from build123d import *


with BuildPart() as part:
    # Эскиз1 → Повернуть1 (revolve)
    with BuildSketch(Plane(origin=(0, 0, 0), x_dir=(1, 0, 0), z_dir=(0, 1, 0)), mode=Mode.PRIVATE) as revolve_1_sk:
        Polygon((5.5, 5), (5.5, 6), (4.5, 6), (4.5, 7), (3.5, 7), (3.5, 8), (6, 8), (6, 10), (3, 10), (3, -10), (6, -10), (6, -8), (3.5, -8), (3.5, -7), (4.5, -7), (4.5, -6), (5.5, -6), (5.5, -5), (6.5, -5), (6.5, -4), (7.5, -4), (7.5, 4), (6.5, 4), (6.5, 5), align=None)
    revolve(revolve_1_sk.sketch.rotate(Axis((0, 0, -10), (0, 0, 1)), 180), axis=Axis((0, 0, -10), (0, 0, 1)))


solid = part.part
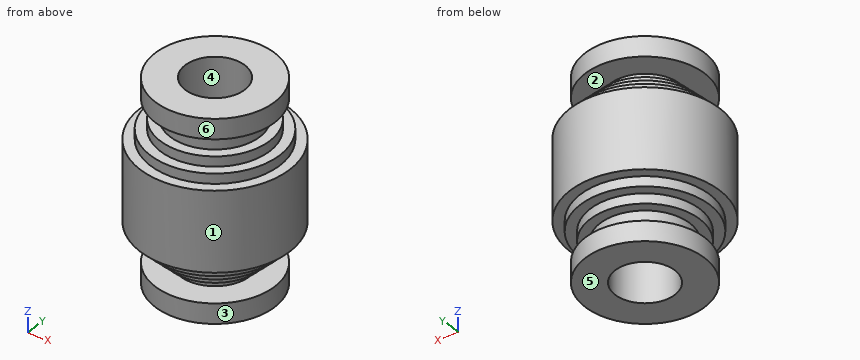
Work out the finished part from the listing and answer in its coordinate system (mm). Face numbers are marked on the shaded views. A direction names the side the tool comes from. Give positions to 0.01 mm unless a question says otherwise; leave off trailing zeros. Order: outer loops, then holes, each group sorted by start corner. A loop starts at its lowest first (then second) coordinate and runs counter-clockwise, first axis right, second up. Notation, with made-up numbers: (36.25, -9) -> (50.25, -9) arc R7 ccw to (50.25, 1) -> close; hole circle Ø10 at (2.5, 26.5). An arc over 180 degrees is marked (long way). Answer as a JSON object with one key per item and string values. Group by question number.
1. Flat-ended cylindrical pins translate along their axes: pin 1 Ø4.5 at (x, y) = (0, 2) entering from -Z; pin 2 Ø1.5 at (y, z) = (-3.5, 3) entering from -X; pin 3 Ø1.5 at (x, z) = (-4.5, 1) entering from +Y; pin 4 Ø3 at (x, z) = (2.5, 8) entering from +Y. Find the tip coordinate at first contact, or state that the pin passes through.
2. A tool of negligible diameter and unlimited length cuts with its end or side. For the marked faces 1, 2 and 3, from which of +Z, -Z, +X, -X, +Y, -Y can it reach the whole face along a straight path? Write none if from no direction.
3. Consider line 1 along Z through (x, y) = (-4.5, 1); line 2 along Y through (x, z) = (0, 2.75); line 3 along Y through (x, z) = (0, 7.25). Determine where each line is inside the solid, lowest interval first. Write a range as [from, to].
4. The mould has two halves that part along X. Classify the marked faces 4, 5 and 6: released by +X, released by -X, zero draft, split by the parting line, or undercut.
5. Section A-A on y = -5.25 is taken. Determine the outline of the cut face in (x, z), plus the area to 3 significant figures.
6. Section B-B on x = 4 is taken. Count the separate pieces of the cut face and the enclosed holes in it, plus the area to 3 significant figures.
7. Section C-C on z = -6.25 is taken. Determine the outline of the cut face in (x, y), plus the area to 3 significant figures.
Result sheet:
{
 "1": {"pin 1": "stops at z = -10", "pin 2": "stops at x = -6.98", "pin 3": "stops at y = 6.5", "pin 4": "stops at y = 5.92"},
 "2": {"face 1": "+Z, -Z", "face 2": "none", "face 3": "-Z"},
 "3": {"line 1": "z = [-10, -8], [-6, 6], [8, 10]", "line 2": "y = [-7.5, -3], [3, 7.5]", "line 3": "y = [-3.5, -3], [3, 3.5]"},
 "4": {"face 4": "undercut", "face 5": "zero draft", "face 6": "split by the parting line"},
 "5": {"outline": "(-5.36, -4) -> (-3.83, -4) -> (-3.83, -5) -> (-1.64, -5) -> (-1.64, -6) -> (1.64, -6) -> (1.64, -5) -> (3.83, -5) -> (3.83, -4) -> (5.36, -4) -> (5.36, 4) -> (3.83, 4) -> (3.83, 5) -> (1.64, 5) -> (1.64, 6) -> (-1.64, 6) -> (-1.64, 5) -> (-3.83, 5) -> (-3.83, 4) -> (-5.36, 4) -> close; (-2.9, -10) -> (2.9, -10) -> (2.9, -8) -> (-2.9, -8) -> close; (-2.9, 8) -> (2.9, 8) -> (2.9, 10) -> (-2.9, 10) -> close", "area": "131 mm^2"},
 "6": {"separate pieces": "3", "enclosed holes": "0", "area": "181 mm^2"},
 "7": {"outline": "circle Ø9 at (0, 0); hole circle Ø6 at (0, 0)", "area": "35.3 mm^2"}
}
